Check sheet for the modelled part. Datum: model origin and axes. Units: mm. Round coordinates to 2 decimals unless told otherwise and drop trailing zeros. Write each loop counter-clockwise with the first axis right and the second up, starting at its lowest first coordinate (ties: lowest second). Pieces come first, ordered by that corner, then holes. Notation, with made-up numbers: M -14,45 L 19,45 A31 ccw 19,71 Z; hole C -20,-22.75 d11. An arc over 180 degrees is marked long. Put each result on its own line as item: value.
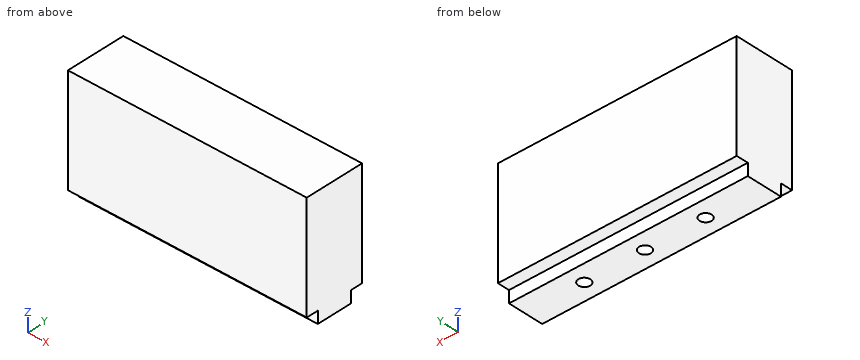
```python
from build123d import *

# Parameters (mm, degrees)
SKICA1_W                 = 10
SKICA1_H                 = 2.5
P_IDAT_VYSUNUT_M1_DEPTH  = 5
SKICA2_W                 = 0.5
SKICA2_H                 = 0.5
ODEBRAT_VYSUNUT_M1_DEPTH = 11
SKICA3_R                 = 0.25
ODEBRAT_VYSUNUT_M2_DEPTH = 1


with BuildPart() as part:
    # Skica1 → Přidat vysunutím1 (new body)
    with BuildSketch(Plane.XY):
        Rectangle(SKICA1_W, SKICA1_H)
    extrude(amount=P_IDAT_VYSUNUT_M1_DEPTH)

    # Skica2 → Odebrat vysunutím1 (cut, through all)
    with BuildSketch(Plane(origin=(5, 0, 0), x_dir=(0, 0, -1), z_dir=(1, 0, 0))):
        with Locations((-0.25, 1)):
            Rectangle(SKICA2_W, SKICA2_H)
        with Locations((-0.25, -1)):
            Rectangle(SKICA2_W, SKICA2_H)
    extrude(amount=-ODEBRAT_VYSUNUT_M1_DEPTH, mode=Mode.SUBTRACT)

    # Skica3 → Odebrat vysunutím2 (cut)
    with BuildSketch(Plane(origin=(0, 0, 0), x_dir=(-1, 0, 0), z_dir=(0, 0, -1))):
        Circle(SKICA3_R)
        with Locations((-2.54, 0)):
            Circle(SKICA3_R)
        with Locations((2.54, 0)):
            Circle(SKICA3_R)
    extrude(amount=-ODEBRAT_VYSUNUT_M2_DEPTH, mode=Mode.SUBTRACT)


solid = part.part
```
1. Cross-section at A-A (y = 0). Enter the section's corners in (x, z), then the cut area to 3 significant figures.
Computed values:
outline: M -5,0 L -2.79,0 L -2.79,1 L -2.29,1 L -2.29,0 L -0.25,0 L -0.25,1 L 0.25,1 L 0.25,0 L 2.29,0 L 2.29,1 L 2.79,1 L 2.79,0 L 5,0 L 5,5 L -5,5 Z
area: 48.5 mm2
2. Scan lines: probe 1 along Y at (x, z) = (-2.54, 0.8); probe 2 along Y at (x, z) = (0, 0.2); probe 3 along Z at (x, y) = (-1, 1.15). Record each from-to range of solid material in increasing order.
Computed values:
probe 1: y = -1.25 to -0.25, 0.25 to 1.25
probe 2: y = -0.75 to -0.25, 0.25 to 0.75
probe 3: z = 0.5 to 5
3. Depth check by flat-ended pin: pin 1 Ø0.6 at (x, z) = (0, 0) entering from -Y. Enter the tip coordinate at first touch or a pass-through.
Computed values:
pin 1: stops at y = -0.75
4. Cross-section at B-B (x = 0). Enter the section's corners in (y, z).
Computed values:
outline: M -1.25,0.5 L -0.75,0.5 L -0.75,0 L -0.25,0 L -0.25,1 L 0.25,1 L 0.25,0 L 0.75,0 L 0.75,0.5 L 1.25,0.5 L 1.25,5 L -1.25,5 Z
